from build123d import *

# Parameters (mm, degrees)
SALIENTE_EXTRUIR1_DEPTH = 5
CROQUIS2_R              = 2
CROQUIS2_R_2            = 4
SALIENTE_EXTRUIR2_DEPTH = 5
CROQUIS3_R              = 2
SALIENTE_EXTRUIR3_DEPTH = 5


with BuildPart() as part:
    # Croquis1 → Saliente-Extruir1 (new body)
    with BuildSketch(Plane.XY):
        with BuildLine():
            Line((-19.085254299, 5.80952381), (20.914745701, 5.80952381))
            ThreePointArc((20.914745701, 5.80952381), (25.914745701, 0.80952381), (20.914745701, -4.19047619))
            Line((20.914745701, -4.19047619), (-19.085254299, -4.19047619))
            ThreePointArc((-19.085254299, -4.19047619), (-24.085254299, 0.80952381), (-19.085254299, 5.80952381))
        make_face()
    extrude(amount=SALIENTE_EXTRUIR1_DEPTH)

    # Croquis2 → Saliente-Extruir2 (add)
    with BuildSketch(Plane.XY.offset(5)):
        with Locations((-19.085254299, 0.80952381)):
            Circle(CROQUIS2_R)
        with Locations((20.914745701, 0.80952381)):
            Circle(CROQUIS2_R_2)
    extrude(amount=SALIENTE_EXTRUIR2_DEPTH)

    # Croquis3 → Saliente-Extruir3 (add)
    with BuildSketch(Plane.XY.offset(10)):
        with Locations((20.914745701, 0.80952381)):
            Circle(CROQUIS3_R)
    extrude(amount=SALIENTE_EXTRUIR3_DEPTH)


solid = part.part
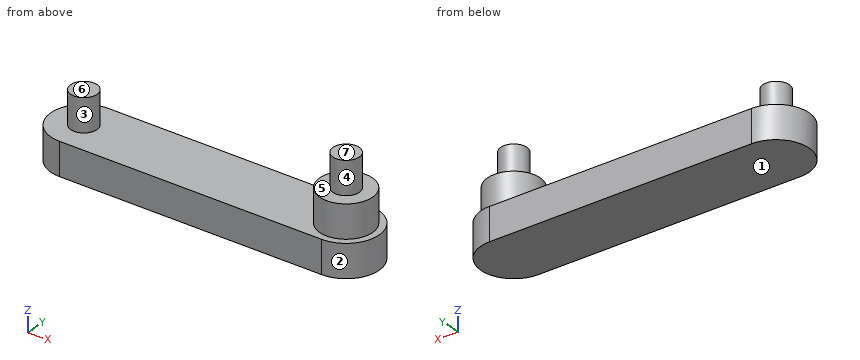
For this review, take the finished solid that the model builds, in its own axes (mm). Face numbers are marked on the shaded views. A direction names the side the tool comes from. Round coordinates to 2 decimals unless told otherwise and drop trailing zeros. Order: outer loops, then holes, each group sorted by start corner. A loop starts at its lowest first (then second) coordinate and runs counter-clockwise, first axis right, second up. Notation, with made-up numbers: M 71,63.25 L 108,63.25 A31 ccw 108,87.25 Z; hole C 5,88.25 d8. An arc over 180 degrees is marked long. Use a Markdown table: item, result. Add a question column.
Item 1: Add section B-B, the plane x = -20.5. Give the boundary of the cut face in (y, z).
Item 2: Add section A-A, the plane y = -0.25. Give the boundary of the cut face in (x, z), then the cut area to 3 significant figures.
Item 3: Mouldability with a two-part tool opening along X and no side actions: class the marked faces 1, 2, 3 and 4 as released by +X, released by -X, zero draft, split by the parting line, or undercut.
Item 4: Add section D-D, the plane z = 6.25. Give the boundary of the cut face in (x, y).
Item 5: Tool access review of the marked faces 5, 6 and 7: name each direction out of +Z, -Z, +X, -X, +Y, -Y from which nothing blocks a thin tool from reaching the whole face with its end or side.
Item 6: Insertion check: pin 1 (4 mm diameter, centred on y = 4.5, z = 8.5, fed in from -X); pin 2 (1.5 mm diameter, centred on y = 1, z = 6.5, fed in from -X); pin 3 (3 mm diameter, centred on x = -18, y = 1, fed in from +Z). Each pin has a flat end and moves straight along its axis. Give the tip position at first contact, or say it passes through.
Item 7: Add section C-C, the plane z = 1.25. Give the boundary of the cut face in (x, y).
Item 8: To check wall thickness, follow line 1 along Z through (x, y) = (-2, 1.5); line 2 along X through (y, z) = (2.5, 8.5); line 3 along Y through (x, z) = (-20, 7.5). State the ranges of each line that lie inside material, in increasing order.
Geometry results:
| question | item | result |
|---|---|---|
| 1 | outline | M -3.99,0 L 5.61,0 L 5.61,5 L 2.22,5 L 2.22,10 L -0.6,10 L -0.6,5 L -3.99,5 Z |
| 2 | outline | M -23.97,0 L 25.8,0 L 25.8,5 L 24.77,5 L 24.77,10 L 22.61,10 L 22.61,15 L 19.22,15 L 19.22,10 L 17.06,10 L 17.06,5 L -17.39,5 L -17.39,10 L -20.78,10 L -20.78,5 L -23.97,5 Z |
| 2 | area | 321 mm² |
| 3 | face 1 | zero draft |
| 3 | face 2 | released by +X |
| 3 | face 3 | undercut |
| 3 | face 4 | split by the parting line |
| 4 | outline | C -19.09,0.81 d4; C 20.91,0.81 d8 |
| 5 | face 5 | +Z |
| 5 | face 6 | +Z, -X, +Y, -Y |
| 5 | face 7 | +Z, +X, -X, +Y, -Y |
| 6 | pin 1 | stops at x = -20.15 |
| 6 | pin 2 | stops at x = -21.09 |
| 6 | pin 3 | stops at z = 10 |
| 7 | outline | M -19.09,-4.19 L 20.91,-4.19 A5 ccw 20.91,5.81 L -19.09,5.81 A5 ccw Z |
| 8 | line 1 | z = 0 to 5 |
| 8 | line 2 | x = -20.15 to -18.02, 17.29 to 24.54 |
| 8 | line 3 | y = -0.97 to 2.59 |
